```python
from build123d import *

# Parameters (mm, degrees)
SKETCH_1_W                   = 300
SKETCH_1_H                   = 50
EXTRUDE_1_DEPTH              = 10
SKETCH_2_W                   = 300
SKETCH_2_H                   = 10.1
SKETCH_2_H_2                 = 9.2
CUT_EXTRUDE_1_DEPTH          = 5
FILLET_1_R                   = 3
CUT_EXTRUDE_START            = -5
SKETCH_10_W                  = 39.8
SKETCH_10_H                  = 15
CUT_EXTRUDE_4_DEPTH          = 145
CUT_EXTRUDE_6_DEPTH          = 51
SKETCH_13_W                  = 50
SKETCH_13_H                  = 35
EXTRUDE_2_DEPTH              = 7.5
HOLE_WIZARD_M4_1_D           = 4.5
HOLE_WIZARD_M4_1_CBORE_D     = 9
HOLE_WIZARD_M4_1_CBORE_DEPTH = 4.1
SKETCH_16_W                  = 6
SKETCH_16_H                  = 6
EXTRUDE_3_DEPTH              = 8
SKETCH_17_R                  = 2.1
CUT_EXTRUDE_7_DEPTH          = 82.5
SKETCH_19_W                  = 6
SKETCH_19_H                  = 6
EXTRUDE_4_DEPTH              = 12
SKETCH_20_R                  = 2.1
CUT_EXTRUDE_9_DEPTH          = 82.5
SKETCH_23_W                  = 34.9
SKETCH_23_H                  = 3
EXTRUDE_9_DEPTH              = 40
HOLE_WIZARD_M4_1_2_D         = 4.5
FILLET_2_R                   = 0.5
SKETCH_27_W                  = 5
SKETCH_27_H                  = 32.4
EXTRUDE_10_DEPTH             = 5
HOLE_WIZARD_M3_1_D           = 2.5
HOLE_WIZARD_M3_1_DEPTH       = 5
EXTRUDE_12_DEPTH             = 5
FILLET_3_R                   = 3
SKETCH_21_R                  = 1.25
FILLET_4_R                   = 10


with BuildPart() as part:
    # 스케치1 → 보스-돌출1 (new body, symmetric)
    with BuildSketch(Plane(origin=(0, 0, 0), x_dir=(1, 0, 0), z_dir=(0, 1, 0))):
        Rectangle(SKETCH_1_W, SKETCH_1_H)
    extrude(amount=EXTRUDE_1_DEPTH, both=True)

    # 스케치2 → 컷-돌출1 (cut)
    with BuildSketch(Plane(origin=(0, 10, 0), x_dir=(1, 0, 0), z_dir=(0, 1, 0))):
        with Locations((0, 11.15)):
            Rectangle(SKETCH_2_W, SKETCH_2_H)
        Rectangle(SKETCH_2_W, SKETCH_2_H_2)
        with Locations((0, -11.15)):
            Rectangle(SKETCH_2_W, SKETCH_2_H)
    extrude(amount=-CUT_EXTRUDE_1_DEPTH, mode=Mode.SUBTRACT)

    # 필렛1
    fillet_1_edges = [part.edges().sort_by_distance(p)[0] for p in [
        (150, 0, 25),
        (-150, 0, 25),
        (-150, 0, -25),
        (150, 0, -25),
    ]]
    fillet(fillet_1_edges, radius=FILLET_1_R)

    # 스케치10 → 컷-돌출4 (cut)
    with BuildSketch(Plane.ZY.offset(150).offset(CUT_EXTRUDE_START)):
        with Locations((0, 2.5)):
            Rectangle(SKETCH_10_W, SKETCH_10_H)
    extrude(amount=-CUT_EXTRUDE_4_DEPTH, mode=Mode.SUBTRACT)

    # 스케치12 → 컷-돌출6 (cut, through all)
    with BuildSketch(Plane.XY.offset(25)):
        Polygon((-40, -10), (-40, -2.5), (0, -2.5), (0, 10), (150, 10), (150, -10), align=None)
    extrude(amount=-CUT_EXTRUDE_6_DEPTH, mode=Mode.SUBTRACT)

    # 스케치13 → 보스-돌출2 (add)
    with BuildSketch(Plane(origin=(0, -10, 0), x_dir=(-1, 0, 0), z_dir=(0, -1, 0))):
        with Locations((65, -42.5)):
            Rectangle(SKETCH_13_W, SKETCH_13_H)
        with Locations((65, 42.5)):
            Rectangle(SKETCH_13_W, SKETCH_13_H)
    extrude(amount=-EXTRUDE_2_DEPTH)

    # Hole Wizard M4 _ _ _ _1 (through all)
    with Locations(Plane(origin=(0, -2.5, 0), x_dir=(1, 0, 0), z_dir=(0, 1, 0))):
        with Locations((-80, 50), (-80, -50)):
            CounterBoreHole(HOLE_WIZARD_M4_1_D / 2, HOLE_WIZARD_M4_1_CBORE_D / 2, HOLE_WIZARD_M4_1_CBORE_DEPTH)

    # 스케치16 → 보스-돌출3 (add)
    with BuildSketch(Plane(origin=(0, -10, 0), x_dir=(-1, 0, 0), z_dir=(0, -1, 0))):
        with Locations((112, -18.5)):
            Rectangle(SKETCH_16_W, SKETCH_16_H)
        with Locations((112, -5)):
            Rectangle(SKETCH_16_W, SKETCH_16_H)
        with Locations((112, 5)):
            Rectangle(SKETCH_16_W, SKETCH_16_H)
        with Locations((112, 18.5)):
            Rectangle(SKETCH_16_W, SKETCH_16_H)
    extrude(amount=EXTRUDE_3_DEPTH)

    # 스케치17 → 컷-돌출7 (cut, through all)
    with BuildSketch(Plane.XY.offset(21.5)):
        with Locations((-112, -14)):
            Circle(SKETCH_17_R)
    extrude(amount=-CUT_EXTRUDE_7_DEPTH, mode=Mode.SUBTRACT)

    # 스케치19 → 보스-돌출4 (add)
    with BuildSketch(Plane.XZ.offset(10)):
        with Locations((-142, 18.5)):
            Rectangle(SKETCH_19_W, SKETCH_19_H)
        with Locations((-142, 4.5)):
            Rectangle(SKETCH_19_W, SKETCH_19_H)
        with Locations((-142, -4.5)):
            Rectangle(SKETCH_19_W, SKETCH_19_H)
        with Locations((-142, -18.5)):
            Rectangle(SKETCH_19_W, SKETCH_19_H)
    extrude(amount=EXTRUDE_4_DEPTH)

    # 스케치20 → 컷-돌출9 (cut, through all)
    with BuildSketch(Plane.XY.offset(21.5)):
        with Locations((-142, -18)):
            Circle(SKETCH_20_R)
    extrude(amount=-CUT_EXTRUDE_9_DEPTH, mode=Mode.SUBTRACT)

    # 스케치23 → 보스-돌출9 (add)
    with BuildSketch(Plane(origin=(-40, 0, 0), x_dir=(0, 0, -1), z_dir=(1, 0, 0))):
        with Locations((-42.55, -4)):
            Rectangle(SKETCH_23_W, SKETCH_23_H)
        with Locations((42.55, -4)):
            Rectangle(SKETCH_23_W, SKETCH_23_H)
    extrude(amount=EXTRUDE_9_DEPTH)

    # Hole Wizard M4 _ _1 2 (through all)
    with Locations(Plane(origin=(0, -2.5, 0), x_dir=(1, 0, 0), z_dir=(0, 1, 0))):
        with Locations((-35, 50), (-5, 50), (-5, -50), (-35, -50)):
            Hole(HOLE_WIZARD_M4_1_2_D / 2)

    # 필렛2
    fillet_2_edges = [part.edges().sort_by_distance(p)[0] for p in [
        (-109, -14, 15.5),
    ]]
    fillet(fillet_2_edges, radius=FILLET_2_R)

    # 스케치27 → 보스-돌출10 (add)
    with BuildSketch(Plane(origin=(0, 5, 0), x_dir=(1, 0, 0), z_dir=(0, 1, 0))):
        with Locations((-147.5, 0)):
            Rectangle(SKETCH_27_W, SKETCH_27_H)
    extrude(amount=EXTRUDE_10_DEPTH)

    # M3 나사 구멍1
    with Locations(Plane(origin=(0, -5, 0), x_dir=(1, 0, 0), z_dir=(0, 1, 0))):
        with Locations((-115, 11.15), (-115, -11.15), (-55, 11.15), (-55, -11.15)):
            Hole(HOLE_WIZARD_M3_1_D / 2, depth=HOLE_WIZARD_M3_1_DEPTH)

    # 스케치34 → 보스-돌출12 (add)
    with BuildSketch(Plane(origin=(0, 10, 0), x_dir=(1, 0, 0), z_dir=(0, 1, 0))):
        Polygon((-150, 25), (-150, -25), (0, -25), (0, -19.9), (-145, -19.9), (-145, 19.9), (0, 19.9), (0, 25), align=None)
    extrude(amount=EXTRUDE_12_DEPTH)

    # 필렛3
    fillet_3_edges = [part.edges().sort_by_distance(p)[0] for p in [
        (-150, 12.5, 25),
        (-150, 12.5, -25),
    ]]
    fillet(fillet_3_edges, radius=FILLET_3_R)

    # 컷-스윕1: sweep along a path in 스케치22
    with BuildLine(Plane(origin=(0, 0, 11.15), x_dir=(-1, 0, 0), z_dir=(0, 0, -1))) as sweep_1_path:
        Line((147.5, -10), (147.5, 9))
        ThreePointArc((147.5, 9), (146.914213562, 10.414213562), (145.5, 11))
        Line((145.5, 11), (144.5, 11))
    # 스케치21 → 컷-스윕1 (sweep, cut)
    with BuildSketch(Plane(origin=(0, -10, 0), x_dir=(-1, 0, 0), z_dir=(0, -1, 0))):
        with Locations((147.5, -11.15)):
            Circle(SKETCH_21_R)
        with Locations((147.5, 11.15)):
            Circle(SKETCH_21_R)
    sweep(path=sweep_1_path.line, mode=Mode.SUBTRACT)

    # 필렛4
    fillet_4_edges = [part.edges().sort_by_distance(p)[0] for p in [
        (-90, -6.25, 60),
        (-90, -6.25, -60),
    ]]
    fillet(fillet_4_edges, radius=FILLET_4_R)


solid = part.part
```
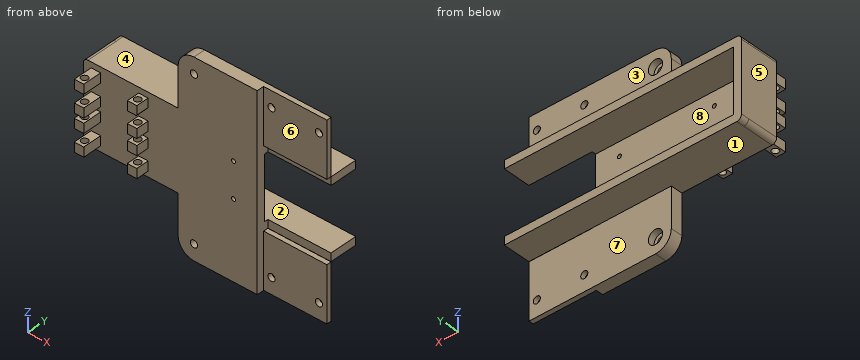
Geometry check sheet. Reference: the model listing, model coordinates, mm. Face numbers are marked on the shaded views. A direction names the side the tool comes from. Coordinates: 2 decimals unless noted, no trailing zeros. Order: outer loops, then holes, each group sorted by start corner. A loop starts at its lowest first (then second) coordinate and runs counter-clockwise, first axis right, second up.
Q1. Draft check along Z on the marked faces 1, 2, 3 and 4. Enter one of: released by +Z, released by -Z, zero draft, split by the parting line, or undercut.
Reply:
face 1: released by -Z
face 2: undercut
face 3: zero draft
face 4: released by +Z
Q2. Sectioned sample at A-A on y = 3.5. Record the cut outline in (x, z), and give its area (3 significant figures).
Reply:
outline: (-150, -22) arc R3 ccw to (-147, -25) - (0, -25) - (0, -19.9) - (-145, -19.9) - (-145, 19.9) - (0, 19.9) - (0, 25) - (-147, 25) arc R3 ccw to (-150, 22) - close; hole circle Ø2.5 at (-147.5, -11.15); hole circle Ø2.5 at (-147.5, 11.15)
area: 1,720 mm2
Q3. Thickness scan on probe 1 along Z at (x, y) = (-80, -3); probe 2 along X at (y, z) = (-4, -50); probe 3 along Z at (x, y) = (-94.5, 2). Record the ranges inside material, lowest first.
Reply:
probe 1: z = -60 to -54.5, -45.5 to -19.9, 19.9 to 45.5, 54.5 to 60
probe 2: x = -90 to -84.5, -75.5 to -37.25, -32.75 to -7.25, -2.75 to 0
probe 3: z = -25 to -19.9, 19.9 to 25
Q4. Depth check by flat-ended pin: pin 1 Ø1.8 at (y, z) = (-13, 20) entering from -X; pin 2 Ø10.5 at (x, z) = (-80, -50) entering from -Y; pin 3 Ø12 at (x, z) = (-134.5, -6) entering from -Y; pin 4 Ø2 at (y, z) = (3.5, -15.5) entering from +X. Enter the tip coordinate at first touch or a pass-through.
Reply:
pin 1: stops at x = -145
pin 2: stops at y = -10
pin 3: stops at y = -22
pin 4: stops at x = -145
Q5. Sectioned sample at C-C on z = -4.5. Record the cut outline in (x, y).
Reply:
outline: (-150, -10) - (-145, -10) - (-145, -22) - (-139, -22) - (-139, -10) - (-115, -10) - (-115, -18) - (-109, -18) - (-109, -10) - (-40, -10) - (-40, -5) - (-145, -5) - (-145, 15) - (-150, 15) - close; hole circle Ø4.2 at (-142, -18); hole circle Ø4.2 at (-112, -14)
Q6. Sectioned sample at B-B on x = -23.5. Record the cut outline in (y, z), and give its area (3 significant figures).
Reply:
outline: (-5.5, -60) - (-2.5, -60) - (-2.5, -25.1) - (-5.5, -25.1) - close; (-5.5, 25.1) - (-2.5, 25.1) - (-2.5, 60) - (-5.5, 60) - close; (-2.5, -25) - (15, -25) - (15, -19.9) - (-2.5, -19.9) - close; (-2.5, 19.9) - (15, 19.9) - (15, 25) - (-2.5, 25) - close
area: 388 mm2
Q7. Sectioned sample at D-D on x = -132. Record the cut outline in (y, z), and give its area (3 significant figures).
Reply:
outline: (-10, -25) - (15, -25) - (15, -19.9) - (-5, -19.9) - (-5, 19.9) - (15, 19.9) - (15, 25) - (-10, 25) - close
area: 454 mm2
Q8. Tool access check on the marked faces 5, 6, 7 and 8. Record the directions out of +Z, -Z, +X, -X, +Y, -Y that give a thin tool (end or side, any length) a straight path to the whole face; none if there is none.
Reply:
face 5: +Z, -Z, -X, +Y, -Y
face 6: +Z, -Z, +X, -Y
face 7: -Z, +X, -X, +Y
face 8: +X, +Y
